Read the model definition and answer for the solid it produces. Units are mm, in the model's axes. A direction names the side the tool comes from. Coordinates: 2 decimals unless noted, no trailing zeros. Write each loop counter-clockwise with the first axis right and the second up, starting at its lowest first coordinate (ties: lowest second). Pieces come first, ordered by that corner, then holes.
(1) Find the intervals of material crossed by probe 1 along X at (y, z) = (14, -9), in increasing order.
(2) Section B-B on y = 16.5 is taken. Write down the section's boundary in (x, z).
(3) Which of the six approach directions +Z, -Z, +X, -X, +Y, -Y give full straight-line access (tool end or side, diameter ignored) to faces 1 (the flat face through (-287, 9.525, -31)), 2 (the flat face through (280.988, 15, -31)), 3 (the flat face through (-4, 0, -31))?
(4) Given pin 1 (12 mm diameter, centred on x = -284, z = -19, fed in from +Y); pin 2 (12 mm diameter, centred on y = 16.5, z = -26, fed in from -X); pin 3 (2 mm diameter, centred on y = 15, z = -48, fed in from +X); pin 4 (3.5 mm diameter, centred on x = 288, z = -27, fed in from +Y) (3 decimals), each flat-ended and moving along its own axis, determine where each tip first touches the part or whether it passes through.
(5) Section A-A on z = -56 is taken. Write down the section's boundary in (x, y) (1 decimal), then the cut area to 3 significant figures.
from build123d import *

# Parameters (mm, degrees)
F0_W     = 584.2
F0_H     = 20.6375
F1_DEPTH = 63.5
F2_W     = 11.1125
F2_H     = 11.1125
F3_DEPTH = 63.501


with BuildPart() as f1:
    # F0 (on Top) → F1 (new body)
    with BuildSketch(Plane.XY):
        with Locations((0, 10.31875)):
            Rectangle(F0_W, F0_H)
    extrude(amount=-F1_DEPTH)

    # F2 (on face) → F3 (cut, through all)
    with BuildSketch(Plane.XY):
        with Locations((286.54375, 15.08125)):
            Rectangle(F2_W, F2_H)
        with Locations((-286.54375, 15.08125)):
            Rectangle(F2_W, F2_H)
    extrude(amount=-F3_DEPTH, mode=Mode.SUBTRACT)


solid = f1.part
Response:
1. probe 1: x = -280.99 to 280.99
2. outline: (-280.99, -63.5) - (280.99, -63.5) - (280.99, 0) - (-280.99, 0) - close
3. face 1: +Z, -Z, -X, +Y
3. face 2: +Z, -Z, +X, +Y
3. face 3: +Z, -Z, +X, -X, -Y
4. pin 1: stops at y = 20.64
4. pin 2: stops at x = -280.99
4. pin 3: stops at x = 280.99
4. pin 4: stops at y = 9.525
5. outline: (-292.1, 0) - (292.1, 0) - (292.1, 9.5) - (281, 9.5) - (281, 20.6) - (-281, 20.6) - (-281, 9.5) - (-292.1, 9.5) - close
5. area: 11,800 mm2
